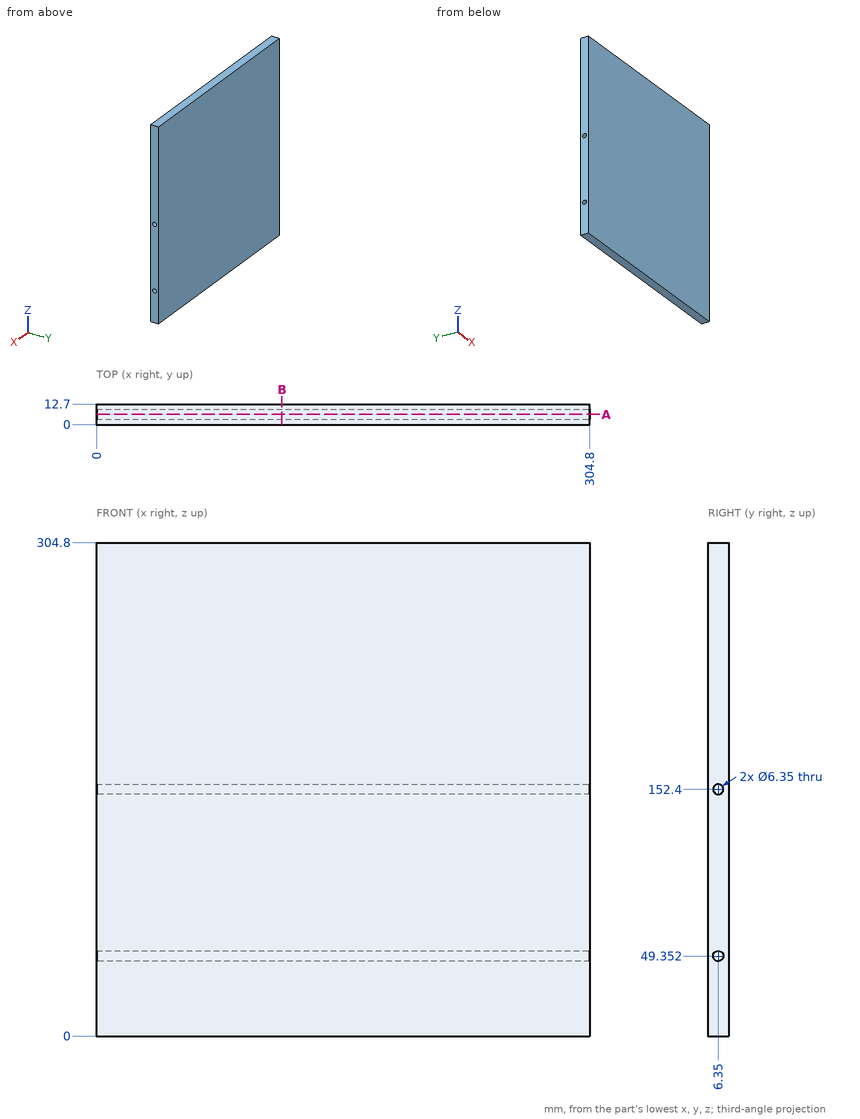
Study the drawing (mm; zero at the part's minimum x, y, z) and answer. Give positions to 0.01 mm unless a question says otherwise; leave off trailing zeros. Loops run counter-clockwise (first coordinate to the right, second up) from the corner with the lowest first, then second, coordinate; pieces in that order, holes last. Notation, with made-up numbers: (34, 21.5) - (40, 21.5) arc R35 ccw to (40, 59.5) - close; hole circle Ø8 at (4, 84.5). An arc over 180 degrees is marked (long way). Answer in a Markdown table with one row per item. Add a question column.
Q1. Consider line 1 along Z through (x, y) = (26.5, 5.75); line 2 along Z through (x, y) = (171, 4.25); line 3 along Y through (x, z) = (179.5, 152.4) (1 decimal). Determine where each line is inside the solid, lowest interval first.
Q2. This flat-tipped pin is pushed along its axis until it touches: P1, Ø7.5, axis at y = 6.35, z = 49.35, coming from the -X side. Where does it stop, or does it pass through?
Q3. The part is cut by section A-A (y = 6.35). Determine the outline of the cut face in (x, z) (1 decimal).
Q4. The part is cut by section B-B (x = 114.5). State how many separate pieces and enclosed holes the cut face has, and give its area (3 significant figures).
Solution:
| question | item | result |
|---|---|---|
| 1 | line 1 | z = 0 to 46.23, 52.47 to 149.28, 155.52 to 304.8 |
| 1 | line 2 | z = 0 to 46.97, 51.73 to 150.02, 154.78 to 304.8 |
| 1 | line 3 | y = 0 to 3.2, 9.5 to 12.7 |
| 2 | P1 | stops at x = 0 |
| 3 | outline | (0, 0) - (304.8, 0) - (304.8, 46.2) - (0, 46.2) - close; (0, 52.5) - (304.8, 52.5) - (304.8, 149.2) - (0, 149.2) - close; (0, 155.6) - (304.8, 155.6) - (304.8, 304.8) - (0, 304.8) - close |
| 4 | separate pieces | 1 |
| 4 | enclosed holes | 2 |
| 4 | area | 3,810 mm² |
